Autodesk Inventor part; units mm, degrees
ref_plane "YZ Plane" through (0, 0, 0) normal (1, 0, 0) x (0, 1, 0)
ref_plane "XZ Plane" through (0, 0, 0) normal (0, 1, 0) x (-1, 0, 0)
ref_plane "XY Plane" through (0, 0, 0) normal (0, 0, 1) x (1, 0, 0)
sketch "Sketch1" plane through (0, 0, 0) normal (0, 1, 0) x (-1, 0, 0)
  line L0 (25, 10) -> (-25, 10)
  line L1 (-25, 10) -> (-25, -10)
  line L2 (-25, -10) -> (25, -10)
  line L3 (25, -10) -> (25, 10)
  line L4 (25, 10) -> (-25, -10) construction
  line L5 (-25, 10) -> (25, -10) construction
  circle A0 centre (-17, 5) radius 3.55
  line L6 (32, 0) -> (-42, 0) construction
  line L7 (0, 26) -> (0, -35) construction
  circle A1 centre (-5, 5) radius 1.6
  circle A2 centre (-17, -5) radius 3.55
  circle A3 centre (-5, -5) radius 1.6
  circle A4 centre (17, 5) radius 3.55
  circle A5 centre (5, 5) radius 1.6
  circle A6 centre (5, -5) radius 1.6
  circle A7 centre (17, -5) radius 3.55
  circle A8 centre (-17, -5) radius 5
  circle A9 centre (-17, 5) radius 5
  circle A10 centre (17, 5) radius 5
  circle A11 centre (17, -5) radius 5
  point P0 (0, 0)
  point P1 (17, 10)
  point P2 (17, 0)
  point P3 (17, -10)
  point P4 (-17, 10)
  point P5 (-17, 0)
  point P6 (-17, -10)
  dimension "d0" = 50
  dimension "d1" = 20
  dimension "d2" = 7.1
  dimension "d3" = 5
  dimension "d4" = 3.2
  dimension "d5" = 12
  dimension "d6" = 10
  dimension "d7" = 10
  dimension "d8" = 10
  dimension "d9" = 10
extrude "Extrusion1" add sketch "Sketch1" along normal blind 5 contours L3 L2 A11 A10 L0 | A10 A11 L2 A8 A9 L0 | A9 A8 L2 L1 L0
extrude "Extrusion2" add sketch "Sketch1" along normal blind 15 contours A10 | A9 | A11 | A8
properties part number "Fix Double Bracket Lifter_3DPrint"
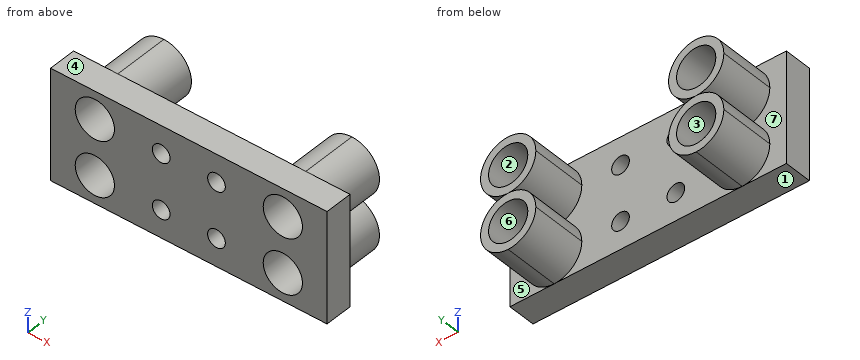
Model file for the job. Use its own axes, mm. Face numbers are marked on the shaded views. A direction names the side the tool comes from. Round coordinates to 2 decimals unless told otherwise and drop trailing zeros. Loops run counter-clockwise (first coordinate to the right, second up) from the corner with the lowest first, then second, coordinate; pieces in that order, holes last.
1. Mould opens along Z. For the marked faces 1, 2, 3 and 4 say: +Z half, -Z half, draft (parallel to the pull), parting line (faces both ways), or undercut.
Check values:
face 1: -Z half
face 2: undercut
face 3: undercut
face 4: +Z half
2. Tool access for the marked faces 5, 6 and 7: list every direction of +Z, -Z, +X, -X, +Y, -Y with a clear straight run to the whole face (end or side of a thin tool).
Check values:
face 5: +X, +Y
face 6: +Y, -Y
face 7: -X, +Y
3. Drop a flat-ended pin along its axis: P1, Ø10, axis at x = 4, z = -7, coming from the +Y side. Give the stop position or say it passes through.
Check values:
P1: stops at y = 5
4. Band-saw the part on D-D, the plane x = -16. List the corners of the cut face in (y, z), and give its area (3 significant figures).
Check values:
outline: (0, -10) - (5, -10) - (5, -9.9) - (15, -9.9) - (15, -8.41) - (0, -8.41) - close; (0, -1.59) - (15, -1.59) - (15, -0.1) - (5, -0.1) - (5, 0.1) - (15, 0.1) - (15, 1.59) - (0, 1.59) - close; (0, 8.41) - (15, 8.41) - (15, 9.9) - (5, 9.9) - (5, 10) - (0, 10) - close
area: 91.6 mm2
5. Band-saw the part on C-C, the plane y = 2.5. Count the separate pieces of the cut face and the enclosed holes in it, and give its area (3 significant figures).
Check values:
separate pieces: 1
enclosed holes: 8
area: 809 mm2
6. Band-saw the part on B-B, the plane x = 5. List the corners of the cut face in (y, z).
Check values:
outline: (0, -10) - (5, -10) - (5, -6.6) - (0, -6.6) - close; (0, -3.4) - (5, -3.4) - (5, 3.4) - (0, 3.4) - close; (0, 6.6) - (5, 6.6) - (5, 10) - (0, 10) - close
7. Wall check: probe 1 along Z at (x, y) = (5, 2.6); probe 2 along X at (y, z) = (2.5, 7.25); probe 3 along Z at (x, y) = (15.5, 14). Give the ranges that are in metal, low to high.
Check values:
probe 1: z = -10 to -6.6, -3.4 to 3.4, 6.6 to 10
probe 2: x = -25 to -19.75, -14.25 to 14.25, 19.75 to 25
probe 3: z = -9.77 to -8.22, -1.78 to -0.23, 0.23 to 1.78, 8.22 to 9.77
